from build123d import *

# Parameters (mm, degrees)
SKETCH1_W           = 171.45
SKETCH1_H           = 25.4
BOSS_EXTRUDE1_DEPTH = 25.4
SKETCH2_W           = 22.86
SKETCH2_H           = 22.86
CUT_EXTRUDE1_DEPTH  = 176.172550646
SKETCH4_R           = 2.413
CUT_EXTRUDE2_DEPTH  = 176.172550646
SKETCH3_R           = 2.413
CUT_EXTRUDE3_DEPTH  = 176.172550646


with BuildPart() as part:
    # Sketch1 → Boss-Extrude1 (new body)
    with BuildSketch(Plane(origin=(0, 0, 0), x_dir=(1, 0, 0), z_dir=(0, 1, 0))):
        with Locations((85.725, 12.7)):
            Rectangle(SKETCH1_W, SKETCH1_H)
    extrude(amount=BOSS_EXTRUDE1_DEPTH)

    # Sketch2 → Cut-Extrude1 (cut, through all)
    with BuildSketch(Plane(origin=(171.45, 0, 0), x_dir=(0, 0, -1), z_dir=(1, 0, 0))):
        with Locations((12.7, 12.7)):
            Rectangle(SKETCH2_W, SKETCH2_H)
    extrude(amount=-CUT_EXTRUDE1_DEPTH, mode=Mode.SUBTRACT)

    # Sketch4 → Cut-Extrude2 (cut, through all)
    with BuildSketch(Plane(origin=(0, 0, -25.4), x_dir=(-1, 0, 0), z_dir=(0, 0, -1))):
        with Locations((-165.1, 12.7)):
            Circle(SKETCH4_R)
        with Locations((-152.4, 12.7)):
            Circle(SKETCH4_R)
        with Locations((-139.7, 12.7)):
            Circle(SKETCH4_R)
        with Locations((-127, 12.7)):
            Circle(SKETCH4_R)
        with Locations((-114.3, 12.7)):
            Circle(SKETCH4_R)
        with Locations((-101.6, 12.7)):
            Circle(SKETCH4_R)
        with Locations((-88.9, 12.7)):
            Circle(SKETCH4_R)
        with Locations((-76.2, 12.7)):
            Circle(SKETCH4_R)
        with Locations((-63.5, 12.7)):
            Circle(SKETCH4_R)
        with Locations((-50.8, 12.7)):
            Circle(SKETCH4_R)
        with Locations((-38.1, 12.7)):
            Circle(SKETCH4_R)
        with Locations((-25.4, 12.7)):
            Circle(SKETCH4_R)
        with Locations((-12.7, 12.7)):
            Circle(SKETCH4_R)
    extrude(amount=-CUT_EXTRUDE2_DEPTH, mode=Mode.SUBTRACT)

    # Sketch3 → Cut-Extrude3 (cut, through all)
    with BuildSketch(Plane(origin=(0, 25.4, 0), x_dir=(1, 0, 0), z_dir=(0, 1, 0))):
        with Locations(Location((6.35, 12.7, 0), (0, 0, 270))):
            Circle(SKETCH3_R)
        with Locations(Location((19.05, 12.7, 0), (0, 0, 270))):
            Circle(SKETCH3_R)
        with Locations(Location((31.75, 12.7, 0), (0, 0, 270))):
            Circle(SKETCH3_R)
        with Locations(Location((44.45, 12.7, 0), (0, 0, 270))):
            Circle(SKETCH3_R)
        with Locations(Location((57.15, 12.7, 0), (0, 0, 270))):
            Circle(SKETCH3_R)
        with Locations(Location((69.85, 12.7, 0), (0, 0, 270))):
            Circle(SKETCH3_R)
        with Locations(Location((82.55, 12.7, 0), (0, 0, 270))):
            Circle(SKETCH3_R)
        with Locations(Location((95.25, 12.7, 0), (0, 0, 270))):
            Circle(SKETCH3_R)
        with Locations(Location((107.95, 12.7, 0), (0, 0, 270))):
            Circle(SKETCH3_R)
        with Locations(Location((120.65, 12.7, 0), (0, 0, 270))):
            Circle(SKETCH3_R)
        with Locations(Location((133.35, 12.7, 0), (0, 0, 270))):
            Circle(SKETCH3_R)
        with Locations(Location((146.05, 12.7, 0), (0, 0, 270))):
            Circle(SKETCH3_R)
        with Locations(Location((158.75, 12.7, 0), (0, 0, 270))):
            Circle(SKETCH3_R)
    extrude(amount=-CUT_EXTRUDE3_DEPTH, mode=Mode.SUBTRACT)


solid = part.part
Input: part model. Units: mm. Frame: model coordinates. A direction names the side the tool comes from. Give positions to 0.01 mm unless a question says otherwise; leave off trailing zeros. Loops run counter-clockwise (first coordinate to the right, second up) from the corner with the lowest first, then second, coordinate; pieces in that order, holes last. Notation, with made-up numbers: M 21.25,12 L 50.25,12 A5 ccw 50.25,16 Z; hole C -40,27 d9. An arc over 180 degrees is marked long. Use one line per item in the form item = value.
1. First-contact query: pin 1 (12 mm diameter, centred on x = 120.5, z = -13.5, fed in from +Y). Flat tip, straight axial feed; report the tip coordinate or a pass-through.
Numbers:
pin_1 = 25.4
2. Section query C-C, the plane z = -20.5. Return the cut outline in (x, y), and give its area (3 significant figures).
Numbers:
outline = M 0,0 L 171.45,0 L 171.45,1.27 L 0,1.27 Z; M 0,24.13 L 171.45,24.13 L 171.45,25.4 L 0,25.4 Z
area = 435 mm²
3. Section query D-D, the plane z = -12.7. Count the separate pieces of the cut face and the enclosed holes in it, and give its area (3 significant figures).
Numbers:
separate_pieces = 28
enclosed_holes = 0
area = 276 mm²
4. Reachability of faces 3 (the face through (87, 10, -24.13)), 4 (the face through (99.37, 11.78, -24.77)) from +Z, -Z, +X, -X, +Y, -Y: full face, straight path, thin tool, end or side. Return the list, or none.
Numbers:
face_3 = +X, -X
face_4 = +Z, -Z
5. Pull-direction query (Z, two-part tool) for faces 1 (the face through (154.81, 12.81, -0.64)), 2 (the face through (8.385, 0.644, -11.403)); classes: released by +Z, released by -Z, zero draft, split by the parting line, or undercut.
Numbers:
face_1 = zero draft
face_2 = undercut
6. Line query: L1, parallel to Z at x = 99.5, y = 10.75; L2, parallel to Y at x = 76.2, z = -0.75; L3, parallel to Y at x = 124, z = -16. Output: solid intervals per line, ascending.
Numbers:
L1 = -25.4 to -24.13, -1.27 to 0
L2 = 0 to 10.29, 15.11 to 25.4
L3 = 0 to 1.27, 24.13 to 25.4
7. Section query B-B, the plane y = 20.25. Return the cut outline in (x, z), and give its area (3 significant figures).
Numbers:
outline = M 0,-25.4 L 171.45,-25.4 L 171.45,-24.13 L 0,-24.13 Z; M 0,-1.27 L 171.45,-1.27 L 171.45,0 L 0,0 Z
area = 435 mm²
8. Section query A-A, the plane x = 165.1. Return the cut outline in (y, z), and give its area (3 significant figures).
Numbers:
outline = M 0,-25.4 L 10.29,-25.4 L 10.29,-24.13 L 1.27,-24.13 L 1.27,-1.27 L 10.29,-1.27 L 10.29,0 L 0,0 Z; M 15.11,-25.4 L 25.4,-25.4 L 25.4,0 L 15.11,0 L 15.11,-1.27 L 24.13,-1.27 L 24.13,-24.13 L 15.11,-24.13 Z
area = 110 mm²
